Autodesk Inventor part; units mm, degrees
ref_plane "YZ Plane" through (0, 0, 0) normal (1, 0, 0) x (0, 1, 0)
ref_plane "XZ Plane" through (0, 0, 0) normal (0, 1, 0) x (-1, 0, 0)
ref_plane "XY Plane" through (0, 0, 0) normal (0, 0, 1) x (1, 0, 0)
sketch "Sketch1" plane through (0, 0, 0) normal (0, 0, 1) x (1, 0, 0)
  line L0 (-10, 8) -> (10, 8)
  line L1 (10, 8) -> (10, -8)
  line L2 (10, -8) -> (-10, -8)
  line L3 (-10, -8) -> (-10, 8)
  line L4 (-10, 8) -> (10, -8) construction
  line L5 (10, 8) -> (-10, -8) construction
  point P0 (0, 0)
  dimension "d0" = 20
  dimension "d1" = 16
extrude "Extrusion1" add sketch "Sketch1" along normal blind 2
sketch "Sketch2" plane through (0, 0, 2) normal (0, 0, 1) x (1, 0, 0)
  line L0 (10, 8) -> (-10, 8)
  line L1 (0, -0.2535) -> (0, 8)
  line L2 (0, 0) -> (0, -7.9613)
  line L3 (-10, -8) -> (10, -8)
  arc A0 (-5.2174, 5.8961) -> (-7.1982, 0.2497) centre (-6, 3) ccw
  arc A1 (7.1982, 0.2497) -> (5.2174, 5.8961) centre (6, 3) ccw
  arc A2 (-5.2174, 5.8961) -> (5.2174, 5.8961) centre (0, 25.2036) ccw
  line L4 (21.5208, 4.9837) -> (21.5208, 0.7791)
  line L5 (-1, -4.7601) -> (-1, -8)
  line L6 (1, -4.7601) -> (1, -8)
  arc A3 (-1, -4.7601) -> (-7.1982, 0.2497) centre (-13.1894, -13.5019) ccw
  arc A4 (7.1982, 0.2497) -> (1, -4.7601) centre (13.1894, -13.5019) ccw
  dimension "d8" = 16
  dimension "d14" = 15.5208
  dimension "d15" = 27.5208
  dimension "d16" = 1
  dimension "d18" = 15
extrude "Extrusion2" add sketch "Sketch2" along normal blind 2
sketch "Sketch3" plane through (0, 0, 4) normal (0, 0, 1) x (1, 0, 0)
  circle A0 centre (-6, 3) radius 1
  line L0 (10, 8) -> (-10, 8)
  circle A1 centre (6, 3) radius 1
  point P0 (0, 0)
  dimension "d21" = 2
  dimension "d22" = 5
extrude "Extrusion3" add sketch "Sketch3" along normal blind 2
sketch "Sketch4" plane through (0, 0, 0) normal (0, 1, 0) x (-1, 0, 0)
  point P0 (0, 0)
sketch "Sketch5" plane through (0, 0, 0) normal (1, 0, 0) x (0, 1, 0)
  point P0 (0, 0)
sketch "Sketch6" plane through (-10, -8, 0) normal (0, -1, 0) x (1, 0, 0)
  line L0 (9, 2) -> (9, 4)
  point P0 (10, 0)
sketch "Sketch7" plane through (-10, -8, 0) normal (0, -1, 0) x (1, 0, 0)
  point P0 (10, 0)
sketch "Sketch8" plane through (0, 0, 0) normal (1, 0, 0) x (0, 1, 0)
  point P0 (0, 0)
sketch "Sketch9" plane through (0, 0, 0) normal (0, 0, 1) x (1, 0, 0)
  point P0 (0, 0)
extrude "Extrusion4" [suppressed]
sketch "Sketch10" plane through (0, 0, 0) normal (0, 1, 0) x (-1, 0, 0)
  point P0 (0, 0)
sketch "Sketch11" plane through (0, 0, 0) normal (0, 1, 0) x (-1, 0, 0)
  point P0 (0, 0)
extrude "Extrusion5" [suppressed]
sketch "Sketch12" plane through (0, 0, 0) normal (1, 0, 0) x (0, 1, 0)
  point P0 (0, 0)
sketch "Sketch13" plane through (0, 0, 0) normal (0, 1, 0) x (-1, 0, 0)
  line L0 (1, 2) -> (1, 4)
  point P0 (0, 0)
sketch "Sketch14" plane through (0, 0, 0) normal (0, 1, 0) x (-1, 0, 0)
  point P0 (0, 0)
extrude "Extrusion6" [suppressed]
sketch "Sketch15" plane through (0, 0, 0) normal (1, 0, 0) x (0, 1, 0)
  arc A0 (-7.985, 19.9445) -> (-7.985, 1.9445) centre (-7.985, 10.9445) ccw
  arc A1 (-7.985, 17.9445) -> (-7.985, 3.9445) centre (-7.985, 10.9445) ccw
  line L0 (-7.985, 1.9445) -> (-7.985, 3.9445)
  arc A2 (-7.985, 17.9445) -> (-7.985, 19.9445) centre (-9.717, 18.9445) ccw
  point P0 (0, 0)
  dimension "d44" = 2
extrude "Extrusion7" add sketch "Sketch15" along normal mid plane 2
properties part number "cad@25"
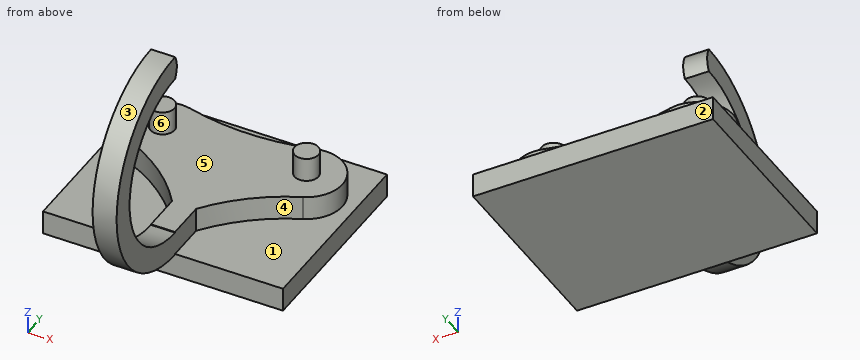
Geometry check sheet. Reference: the model listing, model coordinates, mm. Face numbers are marked on the shaded views. A direction names the side the tool comes from. Round coordinates to 2 decimals unless told otherwise and drop trailing zeros. Write each loop counter-clockwise with the first axis right and the second up, starting at its lowest first coordinate (ties: lowest second). Pieces come first, ordered by that corner, then holes. Notation, with made-up numbers: (62, 49.5) -> (90, 49.5) arc R18 cw to (90, 75.5) -> close; hole circle Ø2 at (-28.75, 31). An arc over 180 degrees is marked (long way). One line per item, written item: value. Start each with the question number.
(1) Access from +Z, -Z, +X, -X, +Y, -Y to the whole of each face (thin tool, end or side, straight path). Record for the marked faces 1 and 2.
(2) Draft check along X on the marked faces 3, 4, 5 and 6. Enter one of: +X half, -X half, draft (parallel to the pull), parting line (faces both ways), or undercut.
(3) Cross-section at C-C, the plane z = 2.5. Record the cut outline in (x, y), and give its area (3 significant figures).
(4) Go/stop test with flat-tipped pins: pin 1 Ø8 at (x, y) = (2.5, -1.5) entering from +Z; pin 2 Ø1 at (x, y) = (6, 3) entering from +Z; pin 3 Ø0.6 at (x, z) = (-2, 0.5) entering from -Y. Record where each tip stops, or that it passes through.
(5) Scan lines: line 1 (Z direction, x = -5, y = 4.5); line 2 (Z direction, x = -8, y = -7); line 3 (X direction, y = -5, z = 2.75). Record each from-to range of solid material in increasing order. Write a range as [from, to].
(6) Cross-section at D-D, the plane x = -5.75. Record the cut outline in (y, z), and give its area (3 significant figures).
(7) Cross-section at A-A, the plane y = 3. Record the cut outline in (x, z), and give its area (3 significant figures).
(8) Cross-section at B-B, the plane x = 3.75. Record the cut outline in (y, z).
Answer:
1. face 1: +Z
1. face 2: +Z, -Z, +X, -X, +Y
2. face 3: draft
2. face 4: +X half
2. face 5: undercut
2. face 6: undercut
3. outline: (-7.2, 0.25) arc R15 cw to (-1, -4.76) -> (-1, -11.1) -> (1, -11.1) -> (1, -4.76) arc R15 cw to (7.2, 0.25) arc R3 ccw to (5.22, 5.9) arc R20 cw to (-5.22, 5.9) arc R3 ccw to start
3. area: 139 mm²
4. pin 1: z = 4
4. pin 2: z = 6
4. pin 3: y = -8
5. line 1: [0, 4]
5. line 2: [0, 2]
5. line 3: [-1, 1]
6. outline: (-8, 0) -> (8, 0) -> (8, 2) -> (5.99, 2) -> (5.99, 4) -> (3.97, 4) -> (3.97, 6) -> (2.03, 6) -> (2.03, 4) -> (-0.48, 4) -> (-0.48, 2) -> (-8, 2) -> close
6. area: 48.8 mm²
7. outline: (-10, 0) -> (10, 0) -> (10, 2) -> (9, 2) -> (9, 4) -> (7, 4) -> (7, 6) -> (5, 6) -> (5, 4) -> (-5, 4) -> (-5, 6) -> (-7, 6) -> (-7, 4) -> (-9, 4) -> (-9, 2) -> (-10, 2) -> close
7. area: 84.0 mm²
8. outline: (-8, 0) -> (8, 0) -> (8, 2) -> (5.56, 2) -> (5.56, 4) -> (-1.84, 4) -> (-1.84, 2) -> (-8, 2) -> close
